The model under review builds one solid part; all positions refer to its coordinate system, in mm. A direction names the side the tool comes from. Round coordinates to 2 decimals unless told otherwise and drop trailing zeros. Loops run counter-clockwise (first coordinate to the right, second up) from the corner with the lowest first, then second, coordinate; pieces in that order, holes last. Notation, with made-up numbers: M 7,64.25 L 17,64.25 A10 ccw 17,68.25 Z; hole C 77,5 d1. An arc over 180 degrees is marked long. Answer as a JSON object with one key per item and string values. Group by question number.
Item 1: The part is to be moulded in two halves that separate along X. For faces 5 (the face through (0, 15, 2)), 6 (the face through (45, 15, 2)), 7 (the face through (23, 15, 2.997)), 8 (the face through (32.5, 1, 2)), say which applies: +X half, -X half, draft (parallel to the pull), parting line (faces both ways), or undercut.
Item 2: Consider section A-A (z = 2). Give the boundary of the cut face in (x, y), and give its area (3 significant figures).
Item 3: Insertion check: P1, Ø0.7, axis at y = 29, z = 2, coming from the -X side; P2, Ø1.2, axis at x = 21.5, z = 1.5, coming from the +Y side; P3, Ø1.2, axis at y = 29.5, z = 2.5, coming from the +X side. Each pin has a flat end and moves straight along its axis. Give the tip position at first contact, or say it passes through.
Item 4: Tool access review of faces 1 (the face through (1, 28, 2)), 2 (the face through (44, 2.3, 2)), 3 (the face through (12.5, 1, 2)), 4 (the face through (42.5, 29, 2)): name each direction out of +Z, -Z, +X, -X, +Y, -Y from which nothing blocks a thin tool from reaching the whole face with its end or side.
Item 5: To check wall thickness, follow line 1 (X direction, y = 29, z = 1.95); line 2 (Y direction, x = 27, z = 1.9). State the ranges of each line that lie inside material, in increasing order.
Item 6: Consider section B-B (x = 23.5). Give the boundary of the cut face in (y, z).
```python
from build123d import *

# Parameters (mm, degrees)
BOSS_EXTRUDE1_DEPTH = 2.3


with BuildPart() as part:
    # Sketch1 → Boss-Extrude1 (new body)
    with BuildSketch(Plane.XY.offset(2.9972)):
        Polygon((0, 2.3), (0, 28), (2.5, 28), (2.5, 30.3), (12.5, 30.3), (12.5, 28), (32.5, 28), (32.5, 30.3), (42.5, 30.3), (42.5, 28), (45, 28), (45, 2.3), (42.5, 2.3), (42.5, 0), (32.5, 0), (32.5, 2.3), (22.5, 2.3), (12.5, 2.3), (12.5, 0), (2.5, 0), (2.5, 2.3), align=None)
    extrude(amount=-BOSS_EXTRUDE1_DEPTH)


solid = part.part
```
Geometry results:
{
 "1": {"face 5": "-X half", "face 6": "+X half", "face 7": "draft", "face 8": "undercut"},
 "2": {"outline": "M 0,2.3 L 2.5,2.3 L 2.5,0 L 12.5,0 L 12.5,2.3 L 32.5,2.3 L 32.5,0 L 42.5,0 L 42.5,2.3 L 45,2.3 L 45,28 L 42.5,28 L 42.5,30.3 L 32.5,30.3 L 32.5,28 L 12.5,28 L 12.5,30.3 L 2.5,30.3 L 2.5,28 L 0,28 Z", "area": "1,250 mm^2"},
 "3": {"P1": "stops at x = 2.5", "P2": "stops at y = 28", "P3": "stops at x = 42.5"},
 "4": {"face 1": "+Z, -Z, -X, +Y", "face 2": "+Z, -Z, +X, -Y", "face 3": "+Z, -Z, -Y", "face 4": "+Z, -Z, +X, +Y"},
 "5": {"line 1": "x = 2.5 to 12.5, 32.5 to 42.5", "line 2": "y = 2.3 to 28"},
 "6": {"outline": "M 2.3,0.7 L 28,0.7 L 28,3 L 2.3,3 Z"}
}
